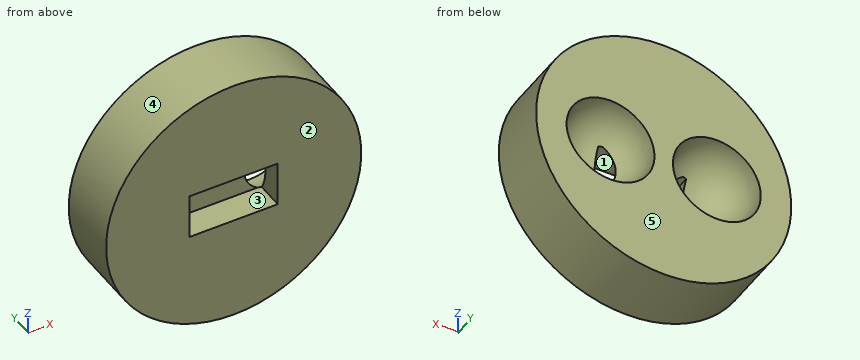
```python
from build123d import *

# Parameters (mm, degrees)
SKETCH2_R           = 9
BOSS_EXTRUDE1_DEPTH = 4.5
SKETCH3_W           = 6.2
SKETCH3_H           = 3.2
CUT_EXTRUDE1_DEPTH  = 2


with BuildPart() as part:
    # Sketch2 → Boss-Extrude1 (new body)
    with BuildSketch(Plane(origin=(0, 0, 0), x_dir=(1, 0, 0), z_dir=(0, 1, 0))):
        with Locations(Location((0, 0, 0), (0, 0, 270))):
            Circle(SKETCH2_R)
    extrude(amount=BOSS_EXTRUDE1_DEPTH)

    # Sketch3 → Cut-Extrude1 (cut)
    with BuildSketch(Plane.XZ):
        Rectangle(SKETCH3_W, SKETCH3_H)
    extrude(amount=-CUT_EXTRUDE1_DEPTH, mode=Mode.SUBTRACT)

    # Sketch4 → Cut-Revolve1 (revolve, cut)
    with BuildSketch(Plane(origin=(0, 4.5, 0), x_dir=(1, 0, 0), z_dir=(0, 1, 0))):
        with BuildLine():
            Line((-3.75, 3.1), (-3.75, -3.1))
            ThreePointArc((-3.75, -3.1), (-6.85, 0), (-3.75, 3.1))
        make_face()
    cut_revolve1 = revolve(axis=Axis((-3.75, 4.5, -3.1), (0, 0, 1)), mode=Mode.SUBTRACT)

    # Mirror1: Cut-Revolve1 across plane
    add(cut_revolve1.mirror(Plane(origin=(0, 0, 0), x_dir=(0, 0, 1), z_dir=(1, 0, 0))), mode=Mode.SUBTRACT)


solid = part.part
```
Input: part model. Units: mm. Frame: model coordinates. Face numbers are marked on the shaded views. A direction names the side the tool comes from. Coordinates: 2 decimals unless noted, no trailing zeros. Order: outer loops, then holes, each group sorted by start corner. A loop starts at its lowest first (then second) coordinate and runs counter-clockwise, first axis right, second up. Notation, with made-up numbers: (49.25, -1.5) - (81.25, -1.5) arc R9 cw to (81.25, 12.5) - close; hole circle Ø4 at (44.25, 4). An arc over 180 degrees is marked (long way). Return JSON: item names as keys, results as strings.
Q1. First-contact query: pin 1 (1.5 mm diameter, centred on y = 1, z = -0.5, fed in from +X); pin 2 (0.6 mm diameter, centred on x = -0.5, y = 1.5, fed in from +Z); pin 3 (0.6 mm diameter, centred on x = -0.5, y = 0.5, fed in from -Z); pin 4 (2 mm diameter, centred on y = 1.5, z = 2.5, fed in from +X). Flat tips, straight axial feed; report the tip coordinate or a pass-through.
The answers:
{"pin 1": "stops at x = 9", "pin 2": "stops at z = 9", "pin 3": "stops at z = -9", "pin 4": "stops at x = 8.87"}
Q2. Cut plane A-A (x = 0). Return loops of the section in (y, z), then the cut area to 3 significant figures.
The answers:
{"outline": "(0, -9) - (4.5, -9) - (4.5, 9) - (0, 9) - (0, 1.6) - (2, 1.6) - (2, -1.6) - (0, -1.6) - close", "area": "74.6 mm2"}
Q3. Cut plane D-D (z = 4.75). Return loops of the section in (x, y), then the cut area to 3 significant figures.
The answers:
{"outline": "(-7.64, 0) - (7.64, 0) - (7.64, 4.5) - (-7.64, 4.5) - close", "area": "68.8 mm2"}
Q4. Cut plane C-C (y = 4.1). Return loops of the section in (x, z), then the cut area to 3 significant figures.
The answers:
{"outline": "circle Ø18 at (0, 0); hole circle Ø6.15 at (-3.75, 0); hole circle Ø6.15 at (3.75, 0)", "area": "195 mm2"}
Q5. Draft query along Z for the marked faces 3, 4 and 5. Return one class per face: +Z half, -Z half, draft (parallel to the pull), parting line (faces both ways), or undercut.
The answers:
{"face 3": "undercut", "face 4": "parting line", "face 5": "draft"}
Q6. Cut plane B-B (z = 0). Return loops of the section in (x, y), then the cut area to 3 significant figures.
The answers:
{"outline": "(-9, 0) - (-3.1, 0) - (-3.1, 1.47) arc R3.1 cw to (-6.85, 4.5) - (-9, 4.5) - close; (-1.92, 2) - (1.92, 2) arc R3.1 cw to (0.65, 4.5) - (-0.65, 4.5) arc R3.1 cw to start; (3.1, 0) - (9, 0) - (9, 4.5) - (6.85, 4.5) arc R3.1 cw to (3.1, 1.47) - close", "area": "39.2 mm2"}
Q7. Access query for the marked faces 1 and 2. Directions: +Z, -Z, +X, -X, +Y, -Y. A direction counts if a zero-diameter tool reaches every point of the face in a straight line with its end or side. Return the directions, or none.
The answers:
{"face 1": "-Y", "face 2": "+Z, -Z, +X, -X, -Y"}
Q8. Ray query, probe 1 along X at (y, z) = (3.5, -1.75); probe 2 along X at (y, z) = (2.45, -0.5); probe 3 along Z at (x, y) = (3, 1.25). Return the intervals inside material, ascending.
The answers:
{"probe 1": "x = -8.83 to -6.11, -1.39 to 1.39, 6.11 to 8.83", "probe 2": "x = -8.99 to -6.02, -1.48 to 1.48, 6.02 to 8.99", "probe 3": "z = -8.49 to -1.6, 1.6 to 8.49"}
